```python
from build123d import *

# Parameters (mm, degrees)
BOSS_EXTRUDE1_DEPTH = 6
SKETCH2_R           = 1.5
CUT_EXTRUDE1_DEPTH  = 104
FILLET1_R           = 10
FILLET2_R           = 3
SKETCH3_R           = 1.5
CUT_EXTRUDE2_DEPTH  = 4


with BuildPart() as part:
    # Sketch1 → Boss-Extrude1 (new body)
    with BuildSketch(Plane.XY):
        Polygon((-157.044043164, 91.385212048), (-157.044043164, 116.385212048), (-56.044043164, 116.385212048), (-56.044043164, 91.385212048), (-60.044043164, 91.385212048), (-60.044043164, 112.385212048), (-153.044043164, 112.385212048), (-153.044043164, 91.385212048), align=None)
    extrude(amount=BOSS_EXTRUDE1_DEPTH)

    # Sketch2 → Cut-Extrude1 (cut)
    with BuildSketch(Plane(origin=(-56.044043164, 0, 0), x_dir=(0, 0, -1), z_dir=(1, 0, 0))):
        with Locations((-3, 94.381633834)):
            Circle(SKETCH2_R)
    extrude(amount=-CUT_EXTRUDE1_DEPTH, mode=Mode.SUBTRACT)

    # Fillet1
    fillet1_edges = [part.edges().sort_by_distance(p)[0] for p in [
        (-157.044043164, 116.385212048, 3),
        (-56.044043164, 116.385212048, 3),
        (-60.044043164, 112.385212048, 3),
        (-153.044043164, 112.385212048, 3),
    ]]
    fillet(fillet1_edges, radius=FILLET1_R)

    # Fillet2
    fillet2_edges = [part.edges().sort_by_distance(p)[0] for p in [
        (-58.044043164, 91.385212048, 6),
        (-58.044043164, 91.385212048, 0),
        (-155.044043164, 91.385212048, 0),
        (-155.044043164, 91.385212048, 6),
    ]]
    fillet(fillet2_edges, radius=FILLET2_R - 0.0001)  # a hair under: the kernel refuses the full size

    # Sketch3 → Cut-Extrude2 (cut)
    with BuildSketch(Plane(origin=(0, 116.385212048, 0), x_dir=(1, 0, 0), z_dir=(0, 1, 0))):
        with Locations(Location((-101.544043164, -3, 0), (0, 0, 270))):
            Circle(SKETCH3_R)
        with Locations(Location((-111.544043164, -3, 0), (0, 0, 90))):
            Circle(SKETCH3_R)
    extrude(amount=-CUT_EXTRUDE2_DEPTH, mode=Mode.SUBTRACT)


solid = part.part
```
Design review of the part built by this model. Coordinates are the model's own, in mm. A direction names the side the tool comes from. Coordinates: 2 decimals unless noted, no trailing zeros. Order: outer loops, then holes, each group sorted by start corner. A loop starts at its lowest first (then second) coordinate and runs counter-clockwise, first axis right, second up.
1) For faces 1 (the cylindrical face through (-62.9, 109.38, 3.04)), 2 (the flat face through (-157.044, 99, 3)), list the 3-axis set-ups (+Z, -Z, +X, -X, +Y, -Y) from which the entire face can be reached by the end or side of a thin tool; tool diameter is ignored.
2) Take a section at B-B, the plane x = -108. Give the boundary of the cut face in (y, z), and give its area (3 significant figures).
3) Wall thickness on line 1 along X through (y, z) = (102.5, 4.85); line 2 along X through (y, z) = (113.5, 3); line 3 along Y through (x, z) = (-116, 2.35): over which ranges is each line inside the solid? List them lowest first.
4) Clearance check with flat-ended pins moving along their axes: pin 1 (2 mm diameter, centred on x = -131, z = 2, fed in from -Y); pin 2 (3.5 mm diameter, centred on x = -101.54, z = 3, fed in from +Y); pin 3 (1 mm diameter, centred on y = 108, z = 2.5, fed in from +X). State where each tip first meets the part, or that it passes through.
5) Take a section at A-A, the plane y = 114.25. Give the boundary of the cut face in (x, z).
6) Mouldability with a two-part tool opening along Z and no side actions: class faces 3 (the cylindrical face through (-58.072, 92.287, 5.145)), 4 (the cylindrical face through (-100.057, 114.413, 2.805)), 5 (the cylindrical face through (-155.02, 93.05, 2.31)), 6 (the cylindrical face through (-155.072, 92.287, 0.855)) as +Z half, -Z half, draft (parallel to the pull), parting line (faces both ways), or undercut.
Returned:
1. face 1: +Z, -Z, -Y
1. face 2: +Z, -Z, -X, +Y, -Y
2. outline: (112.39, 0) - (116.39, 0) - (116.39, 6) - (112.39, 6) - close
2. area: 24.0 mm2
3. line 1: x = -157.04 to -153.04, -60.04 to -56.04
3. line 2: x = -154.07 to -113.04, -110.04 to -103.04, -100.04 to -59.02
3. line 3: y = 112.39 to 116.39
4. pin 1: stops at y = 112.39
4. pin 2: stops at y = 116.39
4. pin 3: stops at x = -56.11
5. outline: (-153.22, 0) - (-59.87, 0) - (-59.87, 6) - (-153.22, 6) - close; hole circle Ø3 at (-111.54, 3); hole circle Ø3 at (-101.54, 3)
6. face 3: +Z half
6. face 4: undercut
6. face 5: undercut
6. face 6: -Z half
